```python
from build123d import *

# Parameters (mm, degrees)
BOSS_EXTRUDE1_DEPTH = 101.6
SKETCH2_R           = 3.048
CUT_EXTRUDE4_DEPTH  = 127


with BuildPart() as part:
    # Sketch1 → Boss-Extrude1 (new body)
    with BuildSketch(Plane(origin=(0, 0, 0), x_dir=(1, 0, 0), z_dir=(0, 1, 0))):
        with BuildLine():
            Line((0.583306021, 0), (5.131693979, 0))
            ThreePointArc((5.131693979, 0), (5.661763503, 0.115908886), (6.095077487, 0.442478269))
            Line((6.095077487, 0.442478269), (8.167782615, 2.855478269))
            ThreePointArc((8.167782615, 2.855478269), (8.358490221, 4.213069524), (7.204399107, 4.953))
            Line((7.204399107, 4.953), (6.0325, 4.953))
            Line((6.0325, 4.953), (6.0325, 6.985))
            Line((6.0325, 6.985), (-0.3175, 6.985))
            Line((-0.3175, 6.985), (-0.3175, 4.953))
            Line((-0.3175, 4.953), (-1.489399107, 4.953))
            ThreePointArc((-1.489399107, 4.953), (-2.643490221, 4.213069524), (-2.452782615, 2.855478269))
            Line((-2.452782615, 2.855478269), (-0.380077487, 0.442478269))
            ThreePointArc((-0.380077487, 0.442478269), (0.053236497, 0.115908886), (0.583306021, 0))
        make_face()
    extrude(amount=BOSS_EXTRUDE1_DEPTH)

    # Sketch2 → Cut-Extrude4 (cut)
    with BuildSketch(Plane(origin=(0, 0, -6.985), x_dir=(-1, 0, 0), z_dir=(0, 0, -1))):
        with Locations((-2.8575, 50.8)):
            Circle(SKETCH2_R)
        with Locations((-2.8575, 88.9)):
            Circle(SKETCH2_R)
        with Locations((-2.8575, 12.7)):
            Circle(SKETCH2_R)
    extrude(amount=-CUT_EXTRUDE4_DEPTH, mode=Mode.SUBTRACT)


solid = part.part
```
Can you work these out from the model? Positions are in its coordinate system, mm. A direction names the side the tool comes from. Coordinates: 2 decimals unless noted, no trailing zeros. Loops run counter-clockwise (first coordinate to the right, second up) from the corner with the lowest first, then second, coordinate; pieces in that order, holes last. Notation, with made-up numbers: (58, 37.25) -> (76, 37.25) arc R8 cw to (76, 41.25) -> close; hole circle Ø9 at (52.5, -38.75). An arc over 180 degrees is marked (long way). Put each result on its own line as item: value. Start each with the question number.
Q1. I want a section at C-C (z = -4). Write out the boundary of the cut face in (x, y).
Q2. I want a section at B-B (x = 3). Write out the boundary of the cut face in (y, z) (3 decimals), plus the area to 3 significant figures.
Q3. If I drill on line 1 (Y direction, x = 0.5, z = -1.5); line 2 (Y direction, x = 5.5, z = -1.75); line 3 (X direction, y = 50.8, z = -4.5), over which ranges is the centre line in solid material (lowest first)? Write a range as [from, to].
Q4. For faces 5 (the face through (6.032, 50, -6)), 6 (the face through (3.254, 53.822, -3.541)), 7 (the face through (-0.318, 50, -6)), which set-ups out of +Z, -Z, +X, -X, +Y, -Y let a thin tool reach every point of the face, with its end or its side?
Q5. Thinking about a two-plate mould opening in Y: for faces 1 (the face through (3, 101.6, -4)), 2 (the face through (3, 70, 0)), 3 (the face through (3, 0, -4)), 4 (the face through (3.254, 15.722, -3.541)), which applies, pulls with the +Y half, pulls with the -Y half, needs draft (parallel to the pull), parting line crosses it, or undercut?
Q6. I'm going to push flat-ended pins straight in: P1, Ø0.6, axis at y = 60.5, z = -6.5, coming from the -X side; P2, Ø0.9, axis at x = 7, y = 38, coming from the -Z side; P3, Ø0.6, axis at y = 54.5, z = -5.5, coming from the +X side; P4, Ø5, axis at x = 2.86, y = 88.9, coming from the +Z side. Where does each tip first touch, or does it pass through?
Q7. I want a section at D-D (y = 75.5). Write out the boundary of the cut face in (x, z) (1 decimal), plus the area to 3 significant figures.
Taken from the geometry:
1. outline: (-2.72, 0) -> (8.43, 0) -> (8.43, 101.6) -> (-2.72, 101.6) -> close; hole circle Ø6.1 at (2.86, 12.7); hole circle Ø6.1 at (2.86, 50.8); hole circle Ø6.1 at (2.86, 88.9)
2. outline: (0, -6.985) -> (9.655, -6.985) -> (9.655, 0) -> (0, 0) -> close; (15.745, -6.985) -> (47.755, -6.985) -> (47.755, 0) -> (15.745, 0) -> close; (53.845, -6.985) -> (85.855, -6.985) -> (85.855, 0) -> (53.845, 0) -> close; (91.945, -6.985) -> (101.6, -6.985) -> (101.6, 0) -> (91.945, 0) -> close
2. area: 582 mm2
3. line 1: y = [0, 10.77], [14.63, 48.87], [52.73, 86.97], [90.83, 101.6]
3. line 2: y = [0, 11.18], [14.22, 49.28], [52.32, 87.38], [90.42, 101.6]
3. line 3: x = [-2.46, -0.19], [5.91, 8.18]
4. face 5: -Z, +X, +Y, -Y
4. face 6: +Z, -Z
4. face 7: -Z, -X, +Y, -Y
5. face 1: pulls with the +Y half
5. face 2: needs draft
5. face 3: pulls with the -Y half
5. face 4: undercut
6. P1: stops at x = -0.32
6. P2: stops at z = -4.95
6. P3: stops at x = 6.03
6. P4: passes through
7. outline: (-2.5, -2.9) arc R1.3 ccw to (-1.5, -5) -> (-0.3, -5) -> (-0.3, -7) -> (6, -7) -> (6, -5) -> (7.2, -5) arc R1.3 ccw to (8.2, -2.9) -> (6.1, -0.4) arc R1.3 ccw to (5.1, 0) -> (0.6, 0) arc R1.3 ccw to (-0.4, -0.4) -> close
7. area: 58.8 mm2
